```python
from build123d import *

# Parameters (mm, degrees)
SKETCH_W        = 105
SKETCH_H        = 120
PAD_DEPTH       = 2.4
SKETCH001_R     = 8.1
SKETCH001_R_2   = 1.1
POCKET_DEPTH    = 5
SKETCH002_W     = 30
SKETCH002_H     = 30
PAD001_DEPTH    = 5
SKETCH003_W     = 20.1
SKETCH003_H     = 20.1
POCKET001_DEPTH = 5
SKETCH004_R     = 10.1
PAD002_DEPTH    = 5
SKETCH005_R     = 5.1
POCKET002_DEPTH = 7.401
SKETCH007_R     = 3.05
POCKET003_DEPTH = 5


with BuildPart() as part:
    # Sketch → Pad (new body)
    with BuildSketch(Plane.XY):
        with Locations((0, -10)):
            Rectangle(SKETCH_W, SKETCH_H)
    extrude(amount=PAD_DEPTH)

    # Sketch001 → Pocket (cut)
    with BuildSketch(Plane.XY.offset(2.4)):
        with Locations((0, -41.5)):
            Circle(SKETCH001_R)
        with Locations((-7.7, -34)):
            Circle(SKETCH001_R_2)
        with Locations((7.7, -34)):
            Circle(SKETCH001_R_2)
        with Locations((-7.7, -49.4)):
            Circle(SKETCH001_R_2)
        with Locations((7.7, -49.4)):
            Circle(SKETCH001_R_2)
    extrude(amount=-POCKET_DEPTH, mode=Mode.SUBTRACT)

    # Sketch002 → Pad001 (new body)
    with BuildSketch(Plane.XY.offset(2.4)):
        with Locations((0, -41.5)):
            Rectangle(SKETCH002_W, SKETCH002_H)
    extrude(amount=PAD001_DEPTH)

    # Sketch003 → Pocket001 (cut)
    with BuildSketch(Plane.XY.offset(7.4)):
        with Locations((0, -41.5)):
            Rectangle(SKETCH003_W, SKETCH003_H)
    extrude(amount=-POCKET001_DEPTH, mode=Mode.SUBTRACT)

    # Sketch004 → Pad002 (new body)
    with BuildSketch(Plane.XY.offset(2.4)):
        with Locations((0, 15)):
            Circle(SKETCH004_R)
    extrude(amount=PAD002_DEPTH)

    # Sketch005 → Pocket002 (cut, through all)
    with BuildSketch(Plane.XY.offset(7.4)):
        with Locations((0, 15)):
            Circle(SKETCH005_R)
    extrude(amount=-POCKET002_DEPTH, mode=Mode.SUBTRACT)

    # Sketch007 → Pocket003 (cut)
    with BuildSketch(Plane.XY.offset(2.4)):
        with Locations((-45, -18)):
            Circle(SKETCH007_R)
        with Locations((45, -18)):
            Circle(SKETCH007_R)
    extrude(amount=-POCKET003_DEPTH, mode=Mode.SUBTRACT)


solid = part.part
```
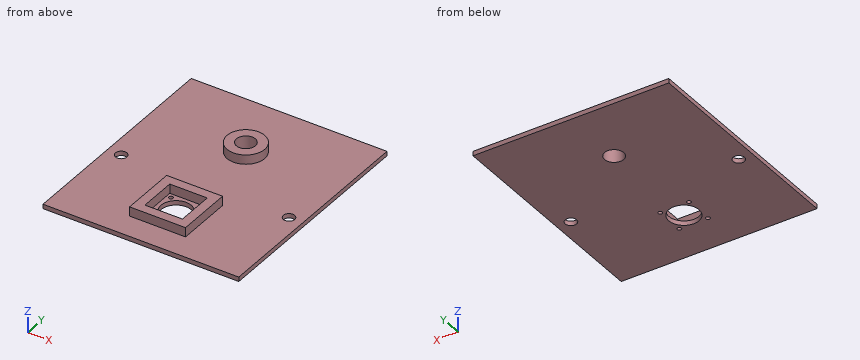
Work out the finished part from the listing and answer in its coordinate system (mm). Give positions to 0.01 mm unless a question says otherwise; leave off trailing zeros. Order: outer loops, then holes, each group sorted by start corner. A loop starts at its lowest first (then second) coordinate and runs counter-clockwise, first axis right, second up. Notation, with made-up numbers: M 46,-39.75 L 50,-39.75 A19 ccw 50,-20.75 Z; hole C -5,53 d2. An arc over 180 degrees is marked long. Return JSON: item names as keys, results as strings.
1) Section A-A, the plane z = 5.75 is taken. Write down the section's boundary in (x, y), plus the area to 3 significant figures.
Resolved:
{"outline": "M -15,-56.5 L 15,-56.5 L 15,-26.5 L -15,-26.5 Z; C 0,15 d20.2; hole M -10.05,-51.55 L 10.05,-51.55 L 10.05,-31.45 L -10.05,-31.45 Z; hole C 0,15 d10.2", "area": "735 mm^2"}
2) Section C-C, the plane y = -41.5 is taken. Write down the section's boundary in (x, z), plus the area to 3 significant figures.
Resolved:
{"outline": "M -52.5,0 L -8.1,0 L -8.1,2.4 L -10.05,2.4 L -10.05,7.4 L -15,7.4 L -15,2.4 L -52.5,2.4 Z; M 8.1,0 L 52.5,0 L 52.5,2.4 L 15,2.4 L 15,7.4 L 10.05,7.4 L 10.05,2.4 L 8.1,2.4 Z", "area": "263 mm^2"}
3) Each of these flat-tipped pins is pushed along its axis until it touches: pin 1 (5 mm diameter, centred on x = 27, y = 7.5, fed in from -Z); pin 2 (4 mm diameter, centred on x = 2, z = 4.5, fed in from +Y); pin 3 (1.5 mm diameter, centred on x = 6.5, z = 4.5, fed in from -Y); pin 4 (3 mm diameter, centred on x = 0, y = -24.5, fed in from +Z). Where does it stop, or does it pass through?
Resolved:
{"pin 1": "z = 0", "pin 2": "y = 25.1", "pin 3": "y = -56.5", "pin 4": "z = 2.4"}
4) Section B-B, the plane x = 0 is taken. Write down the section's boundary in (y, z).
Resolved:
{"outline": "M -70,0 L -49.6,0 L -49.6,2.4 L -51.55,2.4 L -51.55,7.4 L -56.5,7.4 L -56.5,2.4 L -70,2.4 Z; M -33.4,0 L 9.9,0 L 9.9,7.4 L 4.9,7.4 L 4.9,2.4 L -26.5,2.4 L -26.5,7.4 L -31.45,7.4 L -31.45,2.4 L -33.4,2.4 Z; M 20.1,0 L 50,0 L 50,2.4 L 25.1,2.4 L 25.1,7.4 L 20.1,7.4 Z"}
5) Section D-D, the plane x = 45 is taken. Write down the section's boundary in (y, z), plus the area to 3 significant figures.
Resolved:
{"outline": "M -70,0 L -21.05,0 L -21.05,2.4 L -70,2.4 Z; M -14.95,0 L 50,0 L 50,2.4 L -14.95,2.4 Z", "area": "273 mm^2"}
6) Straight lines are drawn through the part: line 1 along Y through (x, z) = (0, 2.5); line 2 along X through (y, z) = (-47.5, 5.75); line 3 along Y through (x, z) = (-2, 4). For each, find the intervals that lie inside material, in ascending order. Write a range as [from, to].
Resolved:
{"line 1": "[-56.5, -51.55], [-31.45, -26.5], [4.9, 9.9], [20.1, 25.1]", "line 2": "[-15, -10.05], [10.05, 15]", "line 3": "[-56.5, -51.55], [-31.45, -26.5], [5.1, 10.31], [19.69, 24.9]"}
